Geometry check sheet. Reference: the model listing, model coordinates, mm. Face numbers are marked on the shaded views. A direction names the side the tool comes from. Round coordinates to 2 decimals unless told otherwise and drop trailing zeros. Loops run counter-clockwise (first coordinate to the right, second up) from the corner with the lowest first, then second, coordinate; pieces in that order, holes last.
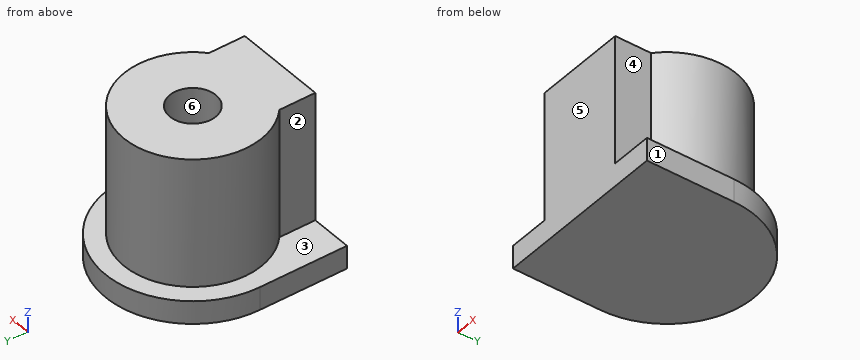
Autodesk Fusion 360 part; units mm, degrees
sketch "Sketch1" plane through (0, 0, 0) normal (0, 0, 1) x (1, 0, 0)
  circle A0 centre (0, 0) radius 3.75
  circle A1 centre (0, 0) radius 1.25
  circle A2 centre (0, 0) radius 4.75
  line L0 (0, 0) -> (0, -4.75)
  line L1 (0, -4.75) -> (2.5, -4.75)
  line L2 (0, -4.75) -> (-2.5, -4.75)
  line L3 (2.5, -4.75) -> (2.5, -2.7951)
  line L4 (-2.5, -4.75) -> (-2.5, -2.7951)
  line L5 (2.5, -4.75) -> (4.75, -4.75)
  line L6 (4.75, -4.75) -> (4.75, 0)
  line L7 (-4.75, 0) -> (-4.75, -4.75)
  line L8 (-4.75, -4.75) -> (-2.5, -4.75)
  dimension "d1" = 7.5
  dimension "d2" = 2.5
  dimension "d3" = 9.5
  dimension "d4" = 2.5
  dimension "d5" = 2.5
  dimension "d10" = 2.25
extrude "Extrude1" add sketch "Sketch1" along normal blind 5 contours A0 | A0 A2 L0 L4 | A0 A2 L0 L3 | A2 L2 L4 | A2 L1 L3
extrude "Extrude2" add sketch "Sketch1" along normal blind 2 contours A1
extrude "Extrude3" add sketch "Sketch1" against normal blind 1.25 contours A1 | A0 | A0 A2 L3 L4 | A0 A2 L0 L4 | A0 A2 L0 L3 | A2 L4 L7 L8 | A2 L2 L4 | A2 L1 L3 | A2 L3 L5 L6
extrude "Extrude4" add 1 faces at (-0.9543, -2.5804, 5) along direction (0, 0, 1) blind 6.444
extrude "Extrude5" cut 1 faces at (-0.9543, -2.5804, 11.444) along direction (0, 0, -1) blind 11.44
extrude "Extrude6" add 1 faces at (-0.9543, -2.5804, 0.004) along direction (0, 0, 1) blind 7
1) Mould release check, pull along X, two halves, no side actions. Record for the marked faces 4, 5 and 6: +X half, -X half, draft (parallel to the pull), parting line (faces both ways), or undercut.
Report:
face 4: +X half
face 5: draft
face 6: undercut
2) Scan lines: line 1 along Y through (x, z) = (0, 5.4); line 2 along Z through (x, y) = (0.5, -1); line 3 along Z through (x, y) = (2.5, 3.5). Record each from-to range of solid material in increasing order.
Report:
line 1: y = -4.75 to -1.25, 1.25 to 3.75
line 2: z = -1.25 to 2
line 3: z = -1.25 to 0
3) Sectioned sample at C-C, the plane z = 6. Record the cut outline in (x, y).
Report:
outline: (-2.5, -4.75) - (2.5, -4.75) - (2.5, -2.8) arc R3.75 ccw (long way) to (-2.5, -2.8) - close; hole circle Ø2.5 at (0, 0)
4) Access from +Z, -Z, +X, -X, +Y, -Y to the whole of each face (thin tool, end or side, straight path). Record for the marked faces 1, 2 and 3.
Report:
face 1: +Z, -Z, +X, +Y, -Y
face 2: +Z, -X, -Y
face 3: +Z
5) Sectioned sample at A-A, the plane y = -2.25. Record the cut outline in (x, z).
Report:
outline: (-4.75, -1.25) - (4.75, -1.25) - (4.75, 0) - (3, 0) - (3, 7) - (-3, 7) - (-3, 0) - (-4.75, 0) - close
6) Sectioned sample at D-D, the plane y = 3.25. Record the cut outline in (x, z), then the cut area to 3 significant figures.
Report:
outline: (-3.46, -1.25) - (3.46, -1.25) - (3.46, 0) - (1.87, 0) - (1.87, 7) - (-1.87, 7) - (-1.87, 0) - (-3.46, 0) - close
area: 34.9 mm2
7) Gauge pin test, flat ends, axial feed: pin 1 (2 mm diameter, centred on y = -3.5, z = 3.5, fed in from -X); pin 2 (0.8 mm diameter, centred on x = 0, y = 0.5, fed in from +Z); pin 3 (0.6 mm diameter, centred on y = -4, z = 2, fed in from +X). Record the tip position at first contact, or that the pin passes through.
Report:
pin 1: stops at x = -2.8
pin 2: stops at z = 2
pin 3: stops at x = 2.5
8) Sectioned sample at B-B, the plane x = 0. Record the cut outline in (y, z), then the cut area to 3 significant figures.
Report:
outline: (-4.75, -1.25) - (4.75, -1.25) - (4.75, 0) - (3.75, 0) - (3.75, 7) - (1.25, 7) - (1.25, 2) - (-1.25, 2) - (-1.25, 7) - (-4.75, 7) - close
area: 58.9 mm2
